Design review of the part built by this model. Coordinates are the model's own, in mm. Round coordinates to 2 decimals unless told otherwise and drop trailing zeros. Order: outer loops, then holes, each group sorted by start corner. A loop starts at its lowest first (then second) coordinate and runs counter-clockwise, first axis right, second up. Notation, with made-up numbers: (44.5, 38) - (101.5, 38) arc R12 cw to (101.5, 59) - close; hole circle Ø2 at (85.5, 26.25). An arc over 180 degrees is marked (long way). Write item = value, one per line.
from build123d import *

# Parameters (mm, degrees)
BASE_FLANGE1_DEPTH     = 1.9
CUT_EXTRUDE4_DEPTH     = 51
CUT_EXTRUDE5_DEPTH     = 71
CUT_EXTRUDE6_START     = 657.08317619
CUT_EXTRUDE6_OUTLINE_W = 45
CUT_EXTRUDE6_OUTLINE_H = 5
CUT_EXTRUDE6_DEPTH     = 6.384307163


# Read off the part's stored shape, not the designer's step: Cut-Extrude6
# Sheet-metal steps are written as plain solids
with BuildPart() as part:
    # Sketch2 → Base-Flange1 (new body)
    with BuildSketch(Plane(origin=(0, 12.879518456, -11.630211804), x_dir=(1, 0, 0), z_dir=(0, 0.7421858097500026, -0.6701941687345042))):
        with BuildLine():
            Line((393.586333182, -753.894678625), (393.586333182, -742.759749552))
            ThreePointArc((393.586333182, -742.759749552), (393.512573412, -742.109852512), (393.295046173, -741.493014958))
            Line((393.295046173, -741.493014958), (348.107032655, -648.432828145))
            Line((348.107032655, -648.432828145), (308.882727398, -648.432828145))
            Line((308.882727398, -648.432828145), (354.876732599, -743.152874081))
            ThreePointArc((354.876732599, -743.152874081), (354.951741991, -743.365576685), (354.977176395, -743.589679113))
            Line((354.977176395, -743.589679113), (354.977176395, -753.894678625))
            Line((354.977176395, -753.894678625), (393.586333182, -753.894678625))
        make_face()
    extrude(amount=BASE_FLANGE1_DEPTH)

    # Sketch7 → Cut-Extrude4 (cut)
    with BuildSketch(Plane(origin=(393.586333182, 0, 0), x_dir=(0, 0, -1), z_dir=(1, 0, 0))):
        Polygon((-546.842488726, 505.418101773), (-542.81093091, 521.489711401), (-552.083782305, 523.815803023), align=None)
    extrude(amount=-CUT_EXTRUDE4_DEPTH, mode=Mode.SUBTRACT)

    # Sketch8 → Cut-Extrude5 (cut)
    with BuildSketch(Plane(origin=(367.203150583, 992.710115794, 1099.346123122), x_dir=(0, 0.9994421284849351, 0.03339808092544755), z_dir=(-1, 0, 0))):
        Polygon((-558.189174553, 593.766016484), (-559.014569405, 618.466070053), (-566.956297266, 616.781727113), (-568.023912054, 608.400656093), align=None)
    extrude(amount=CUT_EXTRUDE5_DEPTH, mode=Mode.SUBTRACT)

    # Cut-Extrude6 outline → Cut-Extrude6 (cut)
    with BuildSketch(Plane(origin=(0, 0, 0), x_dir=(1, 0, 0), z_dir=(0, 0.6701941687345039, 0.7421858097500029)).offset(CUT_EXTRUDE6_START)):
        with Locations((334.5, 18.5)):
            Rectangle(CUT_EXTRUDE6_OUTLINE_W, CUT_EXTRUDE6_OUTLINE_H)
    extrude(amount=CUT_EXTRUDE6_DEPTH, mode=Mode.SUBTRACT)


solid = part.part
1) Clearance check with flat-ended pins moving along their axes: pin 1 Ø12 at (y, z) = (501, 531.5) entering from +X; pin 2 Ø4 at (y, z) = (494, 527) entering from -X; pin 3 Ø5 at (y, z) = (504, 526) entering from -X; pin 4 Ø1.5 at (x, z) = (359, 513.5) entering from -Y. State where each tip first meets the part, or that it passes through.
Findings:
pin_1 = 390.62
pin_2 = through
pin_3 = 347.11
pin_4 = 486.4
2) We need section A-A on x = 335.5. Write out the cut boundary in (y, z).
Findings:
outline = (457.53, 480.79) - (458.94, 479.51) - (485.6, 509.04) - (484.19, 510.31) - close
3) We need section B-B on y = 481.5. Write out the cut boundary in (x, z).
Findings:
outline = (332.53, 504.49) - (371.75, 504.49) - (372.77, 507.33) - (333.55, 507.33) - close
4) To check wall thickness, follow L1, parallel to Z at x = 354.5, y = 491; L2, parallel to Y at x = 323.5, z = 486; L3, parallel to Z at x = 368.5, y = 487.5. State the ranges of each line that lie inside material, in increasing order. Write a range as from..to.
Findings:
L1 = 515.01..517.85
L2 = 462.24..464.8
L3 = 511.14..513.97
